Can you work these out from the model? Positions are in its coordinate system, mm. A direction names the side the tool comes from. Give positions to 0.01 mm unless a question says otherwise; leave off trailing zeros. Order: outer loops, then holes, each group sorted by start corner. A loop starts at its lowest first (then second) coordinate and runs counter-clockwise, first axis right, second up. Notation, with made-up numbers: M 78.5,40 L 95.5,40 A9 ccw 95.5,44 Z; hole C 49,83 d6. An arc over 180 degrees is marked long. Write each question's results on one line, items separated by ' | '.
from build123d import *

# Parameters (mm, degrees)
F1_DEPTH = 25
F4_W     = 32.7306911349
F4_H     = 25
F6_R     = 1.524
F7_W     = 13.5347936116
F7_H     = 8.0888392404
F8_DEPTH = 86.1515196498
F9_W     = 9.5062525943
F9_H     = 25
F12_D    = 5.08


with BuildPart() as f1:
    # F0 (on Front) → F1 (new body, symmetric)
    with BuildSketch(Plane.XZ):
        Polygon((-43.0752597749, 41.8838150799), (-43.0752597749, 0), (0, 0), (43.0752597749, 0), (43.0752597749, 41.8838150799), align=None)
    extrude(amount=F1_DEPTH, both=True)

    # F2 (on face) → F3 (revolve, cut)
    with BuildSketch(Plane.XY.offset(41.8838150799)):
        Polygon((-19.5309855044, 11.865561828), (-26.8544312567, 0), (-12.2075397521, 0), align=None)
    revolve(axis=Axis((0, 0, 41.8838150799), (0, -1, 0)), mode=Mode.SUBTRACT)

    # F4 (on face) → F5 (revolve, cut)
    with BuildSketch(Plane.XY.offset(41.8838150799)):
        with Locations((-16.3653455675, -12.5)):
            Rectangle(F4_W, F4_H)
    revolve(axis=Axis((0, -12.5, 41.8838150799), (0, 1, 0)), mode=Mode.SUBTRACT)

    # F6
    f6_edges = [f1.edges().sort_by_distance(p)[0] for p in [
        (0, 11.865562, 22.35283),
    ]]
    fillet(f6_edges, radius=F6_R)

    # F7 (on face) → F8 (cut, through all)
    with BuildSketch(Plane.YZ.offset(43.0752597749)):
        with Locations((-18.2326031942, 16.8974879198)):
            Rectangle(F7_W, F7_H)
    extrude(amount=-F8_DEPTH, mode=Mode.SUBTRACT)

    # F9 (on face) → F10 (revolve, cut)
    with BuildSketch(Plane.XY.offset(41.8838150799)):
        with Locations((-4.7531262971, 12.5)):
            Rectangle(F9_W, F9_H)
    revolve(axis=Axis((0, 12.5, 41.8838150799), (0, -1, 0)), mode=Mode.SUBTRACT)

    # F12 (through all)
    with Locations(Plane.XZ.offset(25)):
        with Locations((-37.2096933424, 6.1405156739), (37.2096933424, 6.1405156739)):
            Hole(F12_D / 2)


solid = f1.part
(1) I need wall thicknesses on L1, parallel to X at y = -9.5, z = 8; L2, parallel to X at y = -9.5, z = 18.5; L3, parallel to X at y = -12, z = 30. Which ranges of each line are inside material? Lowest first, please. Write a range as from..to.
Data:
L1: x = -43.08..-38.94, -35.48..35.48, 38.94..43.08 | L2: x = -43.08..-22.9, 22.9..43.08 | L3: x = -43.08..-30.5, 30.5..43.08
(2) Imagine slicing it at C-C, the plane y = -1. Write out the boundary of the cut face in (x, z), plus the area to 3 significant figures.
Data:
outline: M -43.08,0 L 43.08,0 L 43.08,41.88 L 32.73,41.88 A32.73 cw -32.73,41.88 L -43.08,41.88 Z; hole C -37.21,6.14 d5.08; hole C 37.21,6.14 d5.08 | area: 1,880 mm2
(3) Will these pins go through, and if not, where does the flat tip stop? P1, Ø13.5, axis at x = -6, z = 37, coming from the -Y side; P2, Ø7, axis at x = 25.5, y = -20, coming from the +Z side; P3, Ø6.5, axis at x = 29, z = 16.5, coming from the -Y side; P4, Ø3, axis at x = -37.21, z = 6.14, coming from the -Y side.
Data:
P1: stops at y = 0 | P2: stops at z = 26.71 | P3: stops at y = -11.47 | P4: passes through
(4) Imagine slicing it at B-B, the plane x = 28.5. Write out the boundary of the cut face in (y, z), plus the area to 3 significant figures.
Data:
outline: M -25,0 L 25,0 L 25,41.88 L 0,41.88 L 0,25.79 L -25,25.79 L -25,20.94 L -11.47,20.94 L -11.47,12.85 L -25,12.85 Z | area: 1,580 mm2
(5) We'd pull the mould along X, two halves only. Please class faces 6 (the face through (-0.47, 9.15, 20.68)), 7 (the face through (-32, -11.465, 17)), 8 (the face through (43.075, 0, 21)): +X half, -X half, draft (parallel to the pull), parting line (faces both ways), or undercut.
Data:
face 6: undercut | face 7: draft | face 8: +X half
(6) Imagine slicing it at A-A, the plane y = -14.5. Write out the boundary of the cut face in (x, z), plus the area to 3 significant figures.
Data:
outline: M -43.08,0 L 43.08,0 L 43.08,12.85 L 15.12,12.85 A32.73 cw -15.12,12.85 L -43.08,12.85 Z; M -43.08,20.94 L -25.15,20.94 A32.73 cw -32.73,41.88 L -43.08,41.88 Z; M 25.15,20.94 L 43.08,20.94 L 43.08,41.88 L 32.73,41.88 A32.73 cw Z; hole C -37.21,6.14 d5.08; hole C 37.21,6.14 d5.08 | area: 1,520 mm2
(7) For faces 1 (the face through (0.72, -12.32, 9.16)), 2 (the face through (-1, -25, 7)), 3 (the face through (34, -18, 20.942)), 4 (the face through (-0.21, 12.68, 32.38)), 5 (the face through (-0.306, 2.781, 27.963)), which set-ups out of +Z, -Z, +X, -X, +Y, -Y let a thin tool reach every point of the face, with its end or its side?
Data:
face 1: +Z, -Y | face 2: +Z, -Z, +X, -X, -Y | face 3: +X, -X, -Y | face 4: +Z, +Y, -Y | face 5: -Y
